```python
from build123d import *

# Parameters (mm, degrees)
SKETCH1_R           = 42.5
BOSS_EXTRUDE1_DEPTH = 119.096016
SKETCH2_R           = 31.251455777
CUT_EXTRUDE1_DEPTH  = 134.403002317
CHAMFER1_SIZE       = 3.853268


with BuildPart() as part:
    # Sketch1 → Boss-Extrude1 (new body)
    with BuildSketch(Plane(origin=(0, 0, 0), x_dir=(1, 0, 0), z_dir=(0, 1, 0))):
        with Locations(Location((0, 0, 0), (0, 0, 270))):
            Circle(SKETCH1_R)
    extrude(amount=BOSS_EXTRUDE1_DEPTH)

    # Sketch2 → Cut-Extrude1 (cut, through all)
    with BuildSketch(Plane(origin=(0, 0, 0), x_dir=(1, 0, 0), z_dir=(0, 1, 0))):
        with Locations(Location((0, 0, 0), (0, 0, 270))):
            Circle(SKETCH2_R)
    extrude(amount=CUT_EXTRUDE1_DEPTH, mode=Mode.SUBTRACT)

    # Chamfer1
    chamfer1_edges = [part.edges().sort_by_distance(p)[0] for p in [
        (0, 0, -42.5),
        (0, 119.096016, -42.5),
        (0, 0, -31.251455777),
        (0, 119.096016, -31.251455777),
    ]]
    chamfer(chamfer1_edges, length=CHAMFER1_SIZE)


solid = part.part
```
Check sheet for the modelled part. Datum: model origin and axes. Units: mm. Round coordinates to 2 decimals unless told otherwise and drop trailing zeros. Loops run counter-clockwise (first coordinate to the right, second up) from the corner with the lowest first, then second, coordinate; pieces in that order, holes last. Notation, with made-up numbers: (-13.5, -23.75) -> (26.5, -23.75) arc R23 ccw to (26.5, -15.75) -> close; hole circle Ø10 at (4, -0.5). An arc over 180 degrees is marked (long way). Write item = value, one per line. Start each with the question number.
1) Release check for a two-part mould opening along Z. For faces 1 (the flat face through (-34.2, 119.096, -8.8)), 2 (the cylindrical face through (-30.51, 58.77, -6.77)), 3 (the conical face through (11.66, 118.91, 37.04)) record: released by +Z, released by -Z, zero draft, split by the parting line, or undercut.
2) Sectioned sample at C-C, the plane y = 98. Record the cut outline in (x, z).
3) Sectioned sample at B-B, the plane z = 0. Record the cut outline in (x, y).
4) Gauge pin test, flat ends, axial feed: pin 1 Ø3 at (y, z) = (72.5, 1.5) entering from +X; pin 2 Ø3 at (y, z) = (31.5, 5) entering from -X; pin 3 Ø1 at (x, y) = (-18.5, 54) entering from -Z. Record the tip position at first contact, or that the pin passes through.
5) Thickness scan on probe 1 along X at (y, z) = (90, 0); probe 2 along X at (y, z) = (37, 9); probe 3 along Z at (x, y) = (-25, 12). Record the ranges inside material, lowest first.
6) Sectioned sample at A-A, the plane x = 0. Record the cut outline in (y, z).
Results are:
q1.face_1 = zero draft
q1.face_2 = undercut
q1.face_3 = split by the parting line
q2.outline = circle Ø85 at (0, 0); hole circle Ø62.5 at (0, 0)
q3.outline = (-42.5, 3.85) -> (-38.65, 0) -> (-35.1, 0) -> (-31.25, 3.85) -> (-31.25, 115.24) -> (-35.1, 119.1) -> (-38.65, 119.1) -> (-42.5, 115.24) -> close; (31.25, 3.85) -> (35.1, 0) -> (38.65, 0) -> (42.5, 3.85) -> (42.5, 115.24) -> (38.65, 119.1) -> (35.1, 119.1) -> (31.25, 115.24) -> close
q4.pin_1 = 42.5
q4.pin_2 = -42.36
q4.pin_3 = -38.5
q5.probe_1 = -42.5 to -31.25, 31.25 to 42.5
q5.probe_2 = -41.54 to -29.93, 29.93 to 41.54
q5.probe_3 = -34.37 to -18.75, 18.75 to 34.37
q6.outline = (0, -38.65) -> (3.85, -42.5) -> (115.24, -42.5) -> (119.1, -38.65) -> (119.1, -35.1) -> (115.24, -31.25) -> (3.85, -31.25) -> (0, -35.1) -> close; (0, 35.1) -> (3.85, 31.25) -> (115.24, 31.25) -> (119.1, 35.1) -> (119.1, 38.65) -> (115.24, 42.5) -> (3.85, 42.5) -> (0, 38.65) -> close
